from build123d import *

# Parameters (mm, degrees)
F1_DEPTH = 0.762
F2_DEPTH = 5.08


with BuildPart() as f1:
    # F0 (on Top) → F1 (new body)
    with BuildSketch(Plane.XY):
        with BuildLine():
            ThreePointArc((-42.241485, 18.570835), (-45.409698, 16.788386), (-47.747653, 14.004744))
            Line((-47.747653, 14.004744), (-43.570547, 8.967645))
            Line((-43.570547, 8.967645), (-47.747653, 3.930546))
            ThreePointArc((-47.747653, 3.930546), (-45.409698, 1.146904), (-42.241485, -0.635545))
            Line((-42.241485, -0.635545), (-38.924205, 3.364703))
            Line((-38.924205, 3.364703), (-35.606926, -0.635545))
            ThreePointArc((-35.606926, -0.635545), (-32.438713, 1.146904), (-30.100758, 3.930546))
            Line((-30.100758, 3.930546), (-34.277864, 8.967645))
            Line((-34.277864, 8.967645), (-30.100758, 14.004744))
            ThreePointArc((-30.100758, 14.004744), (-32.438713, 16.788386), (-35.606926, 18.570835))
            Line((-35.606926, 18.570835), (-38.924205, 14.570586))
            Line((-38.924205, 14.570586), (-42.241485, 18.570835))
        make_face()
    extrude(amount=F1_DEPTH)

    # F0 (on Top) → F2 (join)
    with BuildSketch(Plane.XY):
        with BuildLine():
            ThreePointArc((-35.606926, 18.570835), (-38.924205, 19.127645), (-42.241485, 18.570835))
            Line((-42.241485, 18.570835), (-38.924205, 14.570586))
            Line((-38.924205, 14.570586), (-35.606926, 18.570835))
        make_face()
        with BuildLine():
            ThreePointArc((-30.100758, 3.930546), (-28.764205, 8.967645), (-30.100758, 14.004744))
            Line((-30.100758, 14.004744), (-34.277864, 8.967645))
            Line((-34.277864, 8.967645), (-30.100758, 3.930546))
        make_face()
        with BuildLine():
            Line((-43.570547, 8.967645), (-47.747653, 14.004744))
            ThreePointArc((-47.747653, 14.004744), (-49.084205, 8.967645), (-47.747653, 3.930546))
            Line((-47.747653, 3.930546), (-43.570547, 8.967645))
        make_face()
    extrude(amount=F2_DEPTH)


solid = f1.part
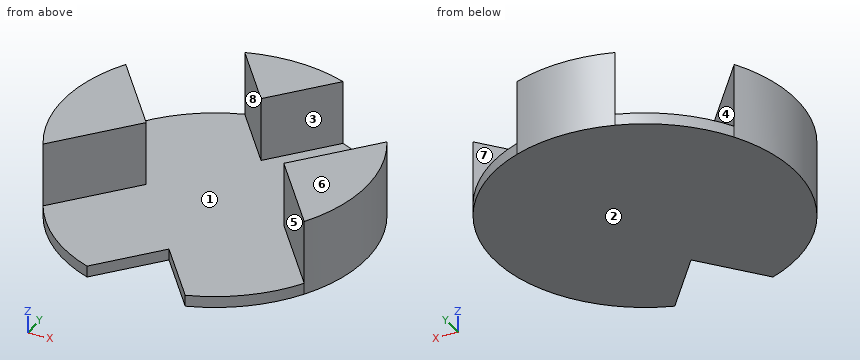
For this review, take the finished solid that the model builds, in its own axes (mm). Face numbers are marked on the shaded views. A direction names the side the tool comes from. Give positions to 0.01 mm unless a question says otherwise; leave off trailing zeros. Order: outer loops, then holes, each group sorted by start corner. A loop starts at its lowest first (then second) coordinate and runs counter-clockwise, first axis right, second up. Notation, with made-up numbers: M 82.25,-0.75 L 109.25,-0.75 A26 ccw 109.25,13.25 Z; hole C -21.75,4.5 d9. An arc over 180 degrees is marked long. Answer in a Markdown table with one row per item. Add a question column.
(1) Consider section A-A on z = 2.5. State the section outline as (x, y) points, and give its area (3 significant figures).
(2) Mouldability with a two-part tool opening along X and no side actions: class the marked faces 6, 7 and 8 as +X half, -X half, draft (parallel to the pull), parting line (faces both ways), or undercut.
(3) Consider section B-B on y = 2.5. State the section outline as (x, z) points.
(4) Consider section D-D on y = 17.25. State the section outline as (x, z) points.
(5) Wall thickness on probe 1 along Z at (x, y) = (-33.25, 1.75); probe 2 along X at (y, z) = (1.5, 0.5); probe 3 along X at (y, z) = (4.5, 1.1): over which ranges is each line inside the solid? List them lowest first. Write a range as [from, to].
(6) For the marked faces 1, 2, 3, 4 and 5, list the 3-axis set-ups (+Z, -Z, +X, -X, +Y, -Y) from which the entire face can be reached by the end or side of a thin tool; tool diameter is ignored.
(7) For pin 1 (2 mm diameter, centred on y = 5.5, z = 4.5, fed in from -X); pin 2 (1.5 mm diameter, centred on x = -46, z = 3.5, fed in from +Y), all flat-tipped, find the tip position at first contact; note any pin that passes through.
(8) Consider section C-C on x = -32. State the section outline as (y, z) points, and give its area (3 significant figures).
Evaluation:
| question | item | result |
|---|---|---|
| 1 | outline | M -47.75,3.93 L -43.57,8.97 L -47.75,14 A10.16 ccw Z; M -42.24,18.57 L -38.92,14.57 L -35.61,18.57 A10.16 ccw Z; M -34.28,8.97 L -30.1,3.93 A10.16 ccw -30.1,14 Z |
| 1 | area | 76.0 mm^2 |
| 2 | face 6 | draft |
| 2 | face 7 | undercut |
| 2 | face 8 | -X half |
| 3 | outline | M -46.76,0 L -39.64,0 L -39.64,0.76 L -46.76,0.76 Z; M -38.21,0 L -31.09,0 L -31.09,0.76 L -38.21,0.76 Z |
| 4 | outline | M -44.81,0 L -33.04,0 L -33.04,0.76 L -36.7,0.76 L -36.7,5.08 L -41.15,5.08 L -41.15,0.76 L -44.81,0.76 Z |
| 5 | probe 1 | z = [0, 0.76] |
| 5 | probe 2 | x = [-45.81, -40.47], [-37.38, -32.04] |
| 5 | probe 3 | x = [-48.05, -47.28], [-30.57, -29.8] |
| 6 | face 1 | +Z |
| 6 | face 2 | -Z, +X, -X, +Y, -Y |
| 6 | face 3 | +Z, +X, -Y |
| 6 | face 4 | +Z, +Y |
| 6 | face 5 | +Z, -Y |
| 7 | pin 1 | stops at x = -48.78 |
| 7 | pin 2 | stops at y = 12.8 |
| 8 | outline | M 1.53,0 L 16.4,0 L 16.4,0.76 L 11.71,0.76 L 11.71,5.08 L 6.22,5.08 L 6.22,0.76 L 1.53,0.76 Z |
| 8 | area | 35.1 mm^2 |
